```python
from build123d import *

# Parameters (mm, degrees)
BOSS_EXTRUDE1_DEPTH      = 3
FILLET4_R                = 21.5
FILLET5_R                = 3.4
FILLET6_R                = 3
F_5_16_CLEARANCE_HOLE1_D = 8.3185
M12_CLEARANCE_HOLE1_D    = 12.1


with BuildPart() as part:
    # Sketch1 → Boss-Extrude1 (new, symmetric)
    with BuildSketch(Plane.XY):
        Polygon((0, 133), (0, 0), (133, 0), (133, 44), (44, 44), (44, 133), align=None)
    extrude(amount=BOSS_EXTRUDE1_DEPTH, both=True)

    # Fillet4
    fillet4_edges = [part.edges().sort_by_distance(p)[0] for p in [
        (133, 44, 0),
        (133, 0, 0),
        (0, 133, 0),
        (44, 133, 0),
    ]]
    fillet(fillet4_edges, radius=FILLET4_R)

    # Fillet5
    fillet5_edges = [part.edges().sort_by_distance(p)[0] for p in [
        (44, 44, 0),
    ]]
    fillet(fillet5_edges, radius=FILLET5_R)

    # Fillet6
    fillet6_edges = [part.edges().sort_by_distance(p)[0] for p in [
        (0, 0, 0),
    ]]
    fillet(fillet6_edges, radius=FILLET6_R)

    # 5/16 Clearance Hole1 (through all)
    with Locations(Plane.XY.offset(3)):
        with Locations((22.5, 111.5), (22.5, 53.7884), (53.7884, 22.5), (111.5, 22.5)):
            Hole(F_5_16_CLEARANCE_HOLE1_D / 2)

    # M12 Clearance Hole1 (through all)
    with Locations(Plane.XY.offset(3)):
        with Locations((22.5, 22.5)):
            Hole(M12_CLEARANCE_HOLE1_D / 2)


solid = part.part
```
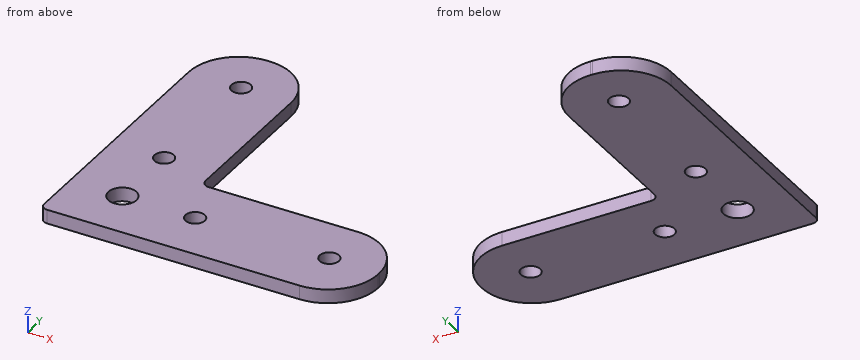
Source: CAD feature listing. Evaluate the final solid. Frame: model axes, mm. Round coordinates to 2 decimals unless told otherwise and drop trailing zeros. Loops run counter-clockwise (first coordinate to the right, second up) from the corner with the lowest first, then second, coordinate; pieces in that order, holes last.
1. Section query A-A on z = 1.95. Output: boundary loops of the cut face in (x, y).
2. Ray query, L1, parallel to X at y = 19, z = -2.5; L2, parallel to Y at x = 88, z = 2.3; L3, parallel to Y at x = 111.5, z = -0.3. Return the intervals inside material, ascending.
3. Section query C-C on x = 79. Output: boundary loops of the cut face in (y, z).
4. Contact query for a flat-ended pin moving along its axis: pin 1 (3 mm diameter, centred on x = 77, z = 0.5, fed in from +Y). Output: stop coordinate, or through.
5. Section query B-B on y = 113.5. Output: boundary loops of the cut face in (x, z).
Answers below:
1. outline: (0, 3) arc R3 ccw to (3, 0) - (111.5, 0) arc R21.5 ccw to (133, 21.5) - (133, 22.5) arc R21.5 ccw to (111.5, 44) - (47.4, 44) arc R3.4 cw to (44, 47.4) - (44, 111.5) arc R21.5 ccw to (22.5, 133) - (21.5, 133) arc R21.5 ccw to (0, 111.5) - close; hole circle Ø12.1 at (22.5, 22.5); hole circle Ø8.32 at (22.5, 53.79); hole circle Ø8.32 at (22.5, 111.5); hole circle Ø8.32 at (53.79, 22.5); hole circle Ø8.32 at (111.5, 22.5)
2. L1: x = 0 to 17.57, 27.43 to 51.54, 56.04 to 109.25, 113.75 to 132.85
2. L2: y = 0 to 44
2. L3: y = 0 to 18.34, 26.66 to 44
3. outline: (0, -3) - (44, -3) - (44, 3) - (0, 3) - close
4. pin 1: stops at y = 44
5. outline: (0.09, -3) - (18.85, -3) - (18.85, 3) - (0.09, 3) - close; (26.15, -3) - (43.91, -3) - (43.91, 3) - (26.15, 3) - close
